Verification items for the finished model (mm, model axes). Face numbers are marked on the shaded views. A direction names the side the tool comes from. Give positions to 0.01 mm unless a question says otherwise; leave off trailing zeros. Loops run counter-clockwise (first coordinate to the right, second up) from the corner with the lowest first, then second, coordinate; pieces in that order, holes last. Notation, with made-up numbers: (56, -23.5) - (99, -23.5) arc R21 cw to (99, 14.5) - close; hole circle Ø5 at (34.25, -25.75). An arc over 180 degrees is marked (long way). Use one line per item in the form item = value.
Autodesk Inventor part; units mm, degrees
ref_plane "YZ Plane" through (0, 0, 0) normal (1, 0, 0) x (0, 1, 0)
ref_plane "XZ Plane" through (0, 0, 0) normal (0, 1, 0) x (-1, 0, 0)
ref_plane "XY Plane" through (0, 0, 0) normal (0, 0, 1) x (1, 0, 0)
sketch "Esquisse1" plane through (0, 0, 0) normal (0, 0, 1) x (1, 0, 0)
  line L0 (-17, 0) -> (-17, 1.5)
  line L1 (-17, 1.5) -> (-14, 1.5)
  line L2 (-14, 1.5) -> (-11.875, 4)
  line L3 (-11.875, 4) -> (-1.875, 4)
  line L4 (-1.875, 4) -> (-1.875, 6)
  line L5 (-1.875, 6) -> (-0.875, 6)
  line L6 (-0.875, 6) -> (-0.875, 5)
  line L7 (5.125, 5) -> (5.125, 6)
  line L8 (5.125, 6) -> (6.125, 6)
  line L9 (6.125, 6) -> (6.125, 4)
  line L10 (6.125, 4) -> (11.875, 4)
  line L11 (11.875, 4) -> (14, 1.5)
  line L12 (14, 1.5) -> (17, 1.5)
  line L13 (17, 1.5) -> (17, 0)
  line L14 (-17, 0) -> (17, 0)
  line L15 (-44.329, 0) -> (0, 0)
  line L16 (-0.875, 5) -> (5.125, 5)
  dimension "d0" = 34
  dimension "d1" = 3
  dimension "d2" = 8
  dimension "d4" = 12
  dimension "d5" = 10
  dimension "d6" = 6
  dimension "d7" = 1
  dimension "d8" = 1
  dimension "d9" = 5.75
  dimension "d10" = 10
  dimension "d12" = 3
  dimension "d13" = 17
  dimension "d17" = 3
revolve "Révolution1" add sketch "Esquisse1" angle 360 about axis through (-44.329, 0, 0) along (1, 0, 0)
equation "\"d8\" = d7"
properties part number "Axe de renvoie" material "Aluminium"
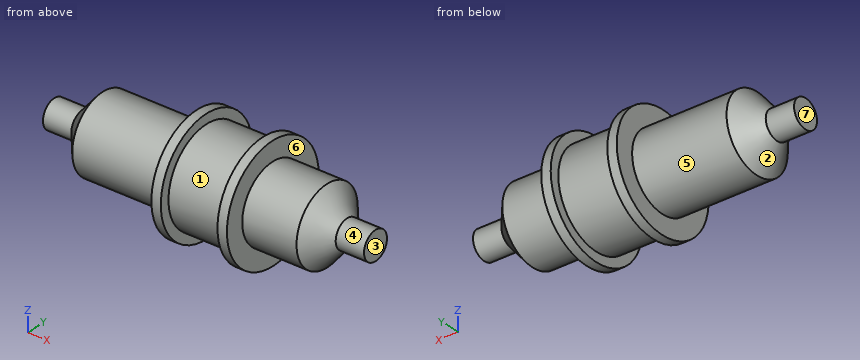
1. Tool access check on the marked faces 5, 6 and 7. Record the directions out of +Z, -Z, +X, -X, +Y, -Y that give a thin tool (end or side, any length) a straight path to the whole face; none if there is none.
Result set:
face_5 = -X
face_6 = +X
face_7 = +Z, -Z, -X, +Y, -Y
2. Section check A-A, the plane z = 0. Record the cut outline in (x, y) (3 decimals).
Result set:
outline = (-17, -1.5) - (-14, -1.5) - (-11.875, -4) - (-1.875, -4) - (-1.875, -6) - (-0.875, -6) - (-0.875, -5) - (5.125, -5) - (5.125, -6) - (6.125, -6) - (6.125, -4) - (11.875, -4) - (14, -1.5) - (17, -1.5) - (17, 1.5) - (14, 1.5) - (11.875, 4) - (6.125, 4) - (6.125, 6) - (5.125, 6) - (5.125, 5) - (-0.875, 5) - (-0.875, 6) - (-1.875, 6) - (-1.875, 4) - (-11.875, 4) - (-14, 1.5) - (-17, 1.5) - close
3. Section check D-D, the plane x = 1. Record the cut outline in (y, z).
Result set:
outline = circle Ø10 at (0, 0)
4. Section check C-C, the plane x = 9. Record the cut outline in (y, z), then the cut area to 3 significant figures.
Result set:
outline = circle Ø8 at (0, 0)
area = 50.3 mm²
5. Draft check along X on the marked faces 1, 2, 3 and 4. Enter one of: released by +X, released by -X, zero draft, split by the parting line, or undercut.
Result set:
face_1 = undercut
face_2 = released by -X
face_3 = released by +X
face_4 = zero draft
6. Scan lines: probe 1 along X at (y, z) = (-5, 2) (3 decimals); probe 2 along Z at (x, y) = (5, -3); probe 3 along Y at (x, z) = (-5.5, -0.25). Record each from-to range of solid material in increasing order.
Result set:
probe_1 = -1.875 to -0.875, 5.125 to 6.125
probe_2 = -4 to 4
probe_3 = -3.99 to 3.99
7. Depth check by flat-ended pin: pin 1 Ø3 at (x, y) = (6, -1.5) entering from -Z; pin 2 Ø1.5 at (x, z) = (7.5, 2) entering from +Y; pin 3 Ø1 at (y, z) = (-3.5, 2.5) entering from +X; pin 4 Ø6 at (x, y) = (10.5, -3.5) entering from -Z. Enter the tip coordinate at first touch or a pass-through.
Result set:
pin_1 = -6
pin_2 = 3.8
pin_3 = 12.04
pin_4 = -3.97
